Geometry check sheet. Reference: the model listing, model coordinates, mm. A direction names the side the tool comes from. Give positions to 0.01 mm unless a question says otherwise; leave off trailing zeros. Write each loop counter-clockwise with the first axis right and the second up, starting at its lowest first coordinate (ties: lowest second). Pieces come first, ordered by that corner, then holes.
(1) Cross-section at B-B (y = -9). Record the boundary of the cut face in (x, z), and give its area (3 significant figures).
(2) Thickness scan on line 1 along Z through (x, y) = (0, -2); line 2 along Z through (x, y) = (-21, 3.5); line 3 along X through (y, z) = (-1.75, 8). Record the ranges inside material, lowest first.
(3) Cross-section at C-C (x = 19.5). Record the boundary of the cut face in (y, z), and give its area (3 significant figures).
(4) Mould release check, pull along X, two halves, no side actions. Record for faces 1 (the cylindrical face through (-0.54, -2.47, 5.56)), 2 (the cylindrical face through (3.39, -2.54, 12.98)), 3 (the cylindrical face through (-3.39, -2.54, 12.98)), 4 (the cylindrical face through (5.34, 0.9, 4.86)): +X half, -X half, draft (parallel to the pull), parting line (faces both ways), or undercut.
(5) Depth check by flat-ended pin: P1, Ø3, axis at y = 10, z = 4, coming from the -X side; P2, Ø2, axis at x = -1.5, z = 10, coming from the +Y side; P3, Ø2, axis at x = 4.5, y = 10, coming from the +Z side. Enter the tip coordinate at first touch or a pass-through.
(6) Tool access check on faces 5 (the cylindrical face through (24.14, 0.28, 3.1)), 6 (the flat face through (0, 0, 11)), 7 (the flat face through (0, -5, 11)). Record the directions out of +Z, -Z, +X, -X, +Y, -Y that give a thin tool (end or side, any length) a straight path to the whole face; none if there is none.
(7) Cross-section at D-D (z = 2.75). Record the boundary of the cut face in (x, y), and give its area (3 significant figures).
(8) Cross-section at A-A (z = 9.5). Record the boundary of the cut face in (x, y).
```python
from build123d import *

# Parameters (mm, degrees)
SKETCH_W     = 50
SKETCH_H     = 40
PAD_DEPTH    = 4
SKETCH001_R  = 2.5
PAD001_DEPTH = 5
FILLET_R     = 3
FILLET001_R  = 6


with BuildPart() as part:
    # Sketch → Pad (new body)
    with BuildSketch(Plane.XY):
        Rectangle(SKETCH_W, SKETCH_H)
    extrude(amount=PAD_DEPTH)

    # Sketch001 → Pad001 (join)
    with BuildSketch(Plane.XZ):
        Polygon((-10, 0), (-4, 14), (4, 14), (10, 0), align=None)
        with Locations((0, 8)):
            Circle(SKETCH001_R, mode=Mode.SUBTRACT)
    extrude(amount=PAD001_DEPTH)

    # Fillet
    fillet_edges = [part.edges().sort_by_distance(p)[0] for p in [
        (-25, 0, 4),
        (0, 20, 4),
        (0, -20, 4),
        (25, 0, 4),
        (-8.285714, -2.5, 4),
        (0, -5, 4),
        (8.285714, -2.5, 4),
        (0, 0, 4),
    ]]
    fillet(fillet_edges, radius=FILLET_R)

    # Fillet001
    fillet001_edges = [part.edges().sort_by_distance(p)[0] for p in [
        (-4, -2.5, 14),
        (4, -2.5, 14),
    ]]
    fillet(fillet001_edges, radius=FILLET001_R)


solid = part.part
```
Reply:
1. outline: (-25, 0) - (25, 0) - (25, 1) arc R3 ccw to (22, 4) - (-22, 4) arc R3 ccw to (-25, 1) - close
1. area: 196 mm2
2. line 1: z = 0 to 5.5, 10.5 to 14
2. line 2: z = 0 to 4
2. line 3: x = -6.57 to -2.5, 2.5 to 6.57
3. outline: (-20, 0) - (20, 0) - (20, 1) arc R3 ccw to (17, 4) - (-17, 4) arc R3 ccw to (-20, 1) - close
3. area: 156 mm2
4. face 1: undercut
4. face 2: +X half
4. face 3: -X half
4. face 4: draft
5. P1: stops at x = -24.6
5. P2: stops at y = 0
5. P3: stops at z = 4
6. face 5: +Z, +X, +Y, -Y
6. face 6: +Z, +X, -X, +Y
6. face 7: +Z, +X, -X, -Y
7. outline: (-24.44, -19.44) - (24.44, -19.44) - (24.44, 19.44) - (-24.44, 19.44) - close
7. area: 1,900 mm2
8. outline: (-5.93, -5) - (-2, -5) - (-2, 0) - (-5.93, 0) - close; (2, -5) - (5.93, -5) - (5.93, 0) - (2, 0) - close
